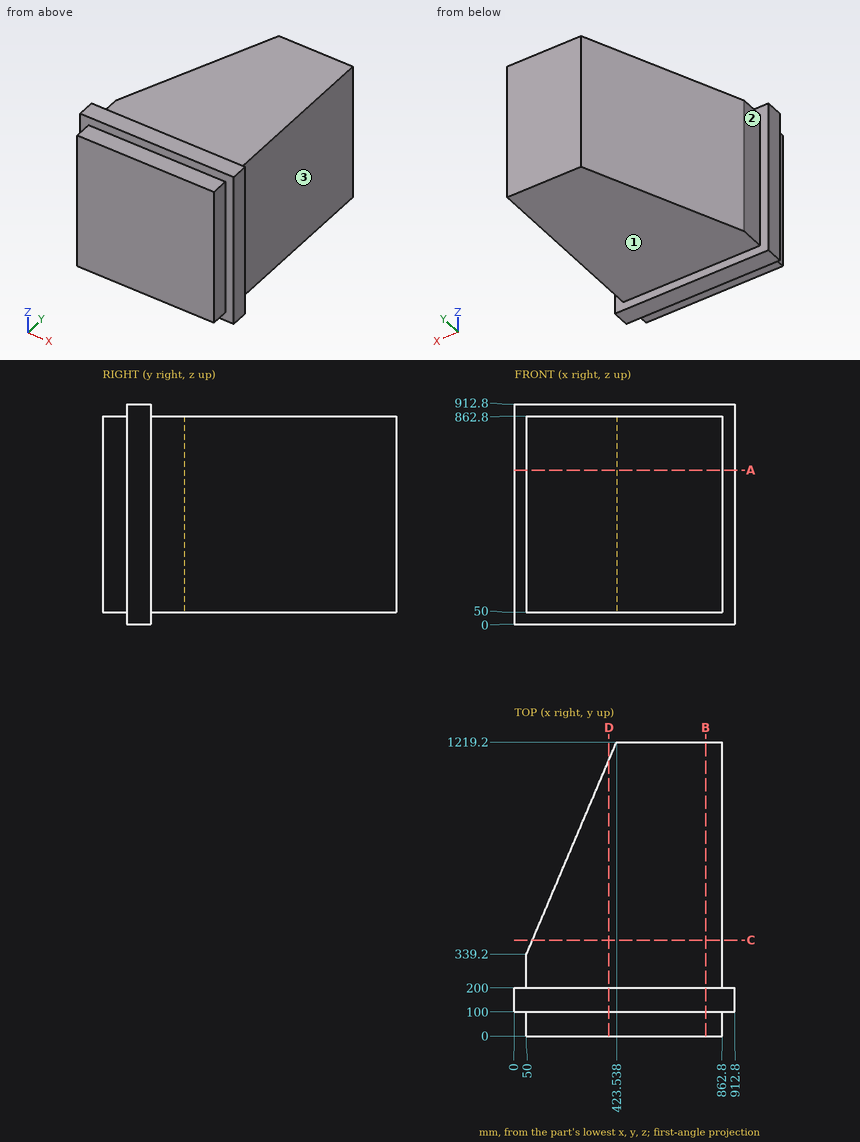
Could you check a few things on this drawing? It's one solid part, dimensions in mm from its lowest x, y, z. A direction names the side the tool comes from. Give positions to 0.01 mm unless a question says otherwise; leave off trailing zeros. Order: outer loops, then holes, each group sorted by start corner. A loop starts at its lowest first (then second) coordinate and runs counter-clockwise, first axis right, second up. Notation, with made-up numbers: (38.25, -2) - (91.25, -2) arc R30 ccw to (91.25, 35) - close; hole circle Ø7 at (73, 0.25). An arc over 180 degrees is marked (long way). One line per item, written item: value. Start each with the question number.
1. Imagine slicing it at B-B on x = 793.5. List the corners of the cut face in (y, z) for me.
2. Imagine slicing it at A-A on z = 638. List the corners of the cut face in (x, y) for me.
3. Imagine slicing it at C-C on y = 397.5. List the corners of the cut face in (x, z) for me, plus the area to 3 significant figures.
4. For P1, Ø10, axis at y = 948.5, z = 415.5, coming from the -X side; P2, Ø6, axis at x = 157.5, z = 194, coming from the +Y side; P3, Ø5, axis at y = 907, z = 629.5, coming from the +X side, each with a flat end and sliding along its axis, tell me the tip position at first contact or that it passes through.
5. If I drill on probe 1 along Z at (x, y) = (349, 1016.5); probe 2 along X at (y, z) = (377, 590) (1 decimal), over which ranges is the centre line in solid material (lowest first)?
6. Imagine slicing it at D-D on x = 392. List the corners of the cut face in (y, z) for me, plus the area to 3 significant figures.
7. For the marked faces 1, 2 and 3, which set-ups out of +Z, -Z, +X, -X, +Y, -Y let a thin tool reach every point of the face, with its end or its side?
Values:
1. outline: (0, 50) - (100, 50) - (100, 0) - (200, 0) - (200, 50) - (1219.2, 50) - (1219.2, 862.8) - (200, 862.8) - (200, 912.8) - (100, 912.8) - (100, 862.8) - (0, 862.8) - close
2. outline: (0, 100) - (50, 100) - (50, 0) - (862.8, 0) - (862.8, 100) - (912.8, 100) - (912.8, 200) - (862.8, 200) - (862.8, 1219.2) - (423.54, 1219.2) - (50, 339.2) - (50, 200) - (0, 200) - close
3. outline: (74.75, 50) - (862.8, 50) - (862.8, 862.8) - (74.75, 862.8) - close
3. area: 641,000 mm²
4. P1: x = 306.51
4. P2: y = 599.52
4. P3: x = 862.8
5. probe 1: 50 to 862.8
5. probe 2: 66 to 862.8
6. outline: (0, 50) - (100, 50) - (100, 0) - (200, 0) - (200, 50) - (1144.9, 50) - (1144.9, 862.8) - (200, 862.8) - (200, 912.8) - (100, 912.8) - (100, 862.8) - (0, 862.8) - close
6. area: 941,000 mm²
7. face 1: -Z, +X, -X, +Y
7. face 2: +Z, -Z, -X, +Y
7. face 3: +Z, -Z, +X, +Y
